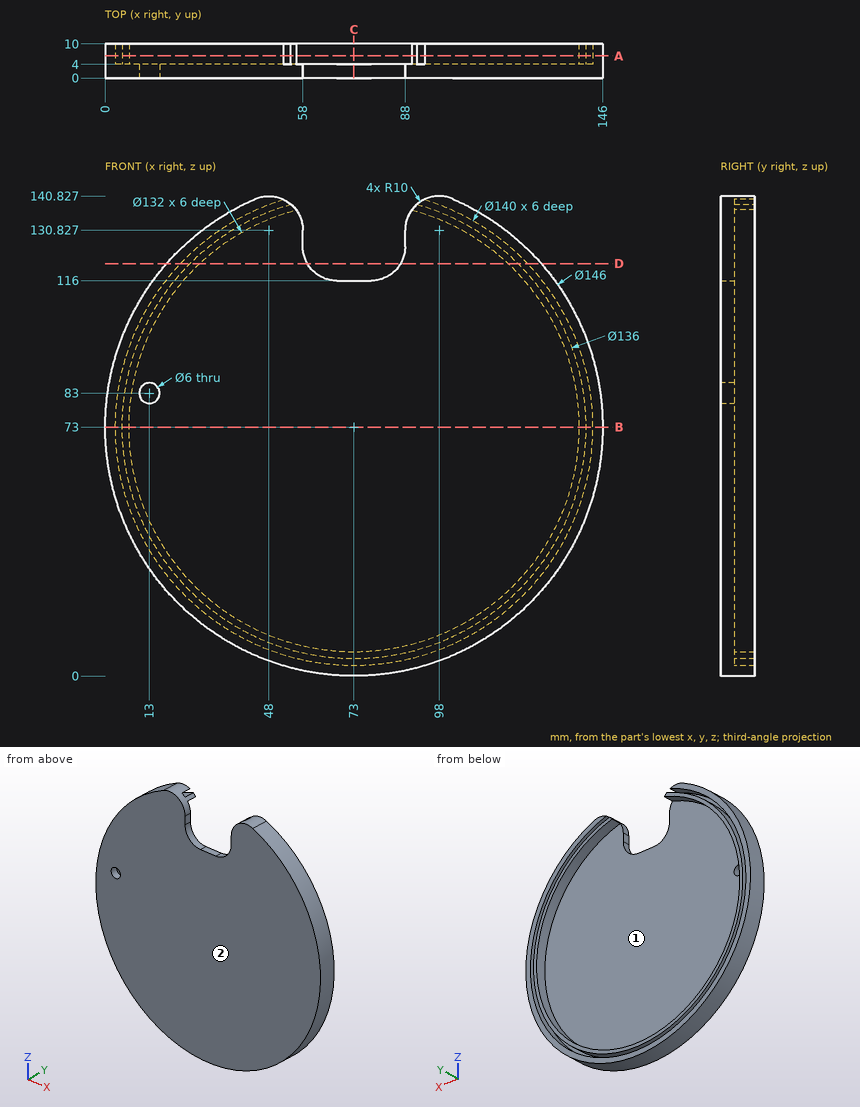
Drawing for the job (mm, zero at the part's lowest x, y, z). Round coordinates to 2 decimals unless told otherwise and drop trailing zeros. Order: outer loops, then holes, each group sorted by start corner. A loop starts at its lowest first (then second) coordinate and runs counter-clockwise, first axis right, second up. Notation, with made-up numbers: M -20,7 L 36,7 A29 ccw 36,28 Z; hole C 63,37 d1. An arc over 180 degrees is marked long. Use one line per item in the form item = value.
Q1. Saw through at B-B on z = 73. Give the cut face in (x, y), then the cut area to 3 significant figures.
Recorded:
outline = M 0,0 L 146,0 L 146,10 L 143,10 L 143,4 L 141,4 L 141,10 L 139,10 L 139,4 L 7,4 L 7,10 L 5,10 L 5,4 L 3,4 L 3,10 L 0,10 Z
area = 644 mm^2
Q2. Flat gauge pins, fed straight in: P1, Ø2, axis at y = 2.5, z = 28.5, coming from the -X side; P2, Ø4.5, axis at x = 71, y = 2.5, coming from the +Z side; P3, Ø1, axis at x = 25.5, y = 3.5, coming from the -Z side; P4, Ø5.5, axis at x = 13, z = 83, coming from the -Y side. Where does each tip first touch, or does it go through?
Recorded:
P1 = 14.38
P2 = 116
P3 = 17.14
P4 = through
Q3. Probe L1, parallel to X at y = 7.1, z = 73; L2, parallel to Z at x = 125, y = 7 (1 decimal); L3, parallel to Z at x = 40, y = 7 (1 decimal). List the from-to ranges inside material, lowest first.
Recorded:
L1 = 0 to 3, 5 to 7, 139 to 141, 143 to 146
L2 = 21.8 to 26.1, 29.2 to 32.4, 113.6 to 116.8, 119.9 to 124.2
L3 = 7.9 to 11.3, 13.5 to 15.8, 130.2 to 132.5, 134.7 to 138.1
Q4. Two-plate mould, pull along X, no slides. Class the marked faces 1 and 2: +X half, -X half, draft (parallel to the pull), parting line (faces both ways), or undercut.
Recorded:
face_1 = undercut
face_2 = draft
Q5. Saw through at C-C on x = 73. Give the cut face in (y, z).
Recorded:
outline = M 0,0 L 10,0 L 10,3 L 4,3 L 4,5 L 10,5 L 10,7 L 4,7 L 4,116 L 0,116 Z
Q6. Saw through at D-D on z = 121. Give the cut face in (x, y), then the cut area to 3 significant figures.
Recorded:
outline = M 18,0 L 59.34,0 L 59.34,4 L 27.7,4 L 27.7,10 L 24.83,10 L 24.83,4 L 22.05,4 L 22.05,10 L 18,10 Z; M 86.66,0 L 128,0 L 128,10 L 123.95,10 L 123.95,4 L 121.17,4 L 121.17,10 L 118.3,10 L 118.3,4 L 86.66,4 Z
area = 414 mm^2
Q7. Saw through at A-A on y = 6.5. Give the cut face in (x, z).
Recorded:
outline = M 44.03,140.01 A73 ccw long 101.97,140.01 A10 ccw 93.72,139.86 A70 cw long 52.28,139.86 A10 ccw Z; M 54.49,138.43 A68 ccw long 91.51,138.43 A10 ccw 89.97,136.78 A66 cw long 56.03,136.78 A10 ccw Z
